from build123d import *

# Parameters (mm, degrees)
F3_DEPTH = 9
F4_SIZE  = 1


with BuildPart() as f1:
    # F0 (on Top) → F1 (revolve)
    with BuildSketch(Plane.XY):
        Polygon((-4, 0), (0, 0), (0, 41), (-6.5, 41), (-6.5, 30), (-4, 30), align=None)
    revolve(axis=Axis((0, 20.5, 0), (0, 1, 0)))

    # F2 (on face) → F3 (cut)
    with BuildSketch(Plane(origin=(0, 41, 0), x_dir=(-1, 0, 0), z_dir=(0, 1, 0))):
        Polygon((-3.255243, -1.184649), (-0.601686, -3.411448), (2.653557, -2.226799), (3.255243, 1.184649), (0.601686, 3.411448), (-2.653557, 2.226799), align=None)
    extrude(amount=-F3_DEPTH, mode=Mode.SUBTRACT)

    # F4
    f4_edges = [f1.edges().sort_by_distance(p)[0] for p in [
        (6.5, 41, 0),
    ]]
    chamfer(f4_edges, length=F4_SIZE)


solid = f1.part
Build history of the part. All positions in model axes, mm. A direction names the side the tool comes from. Coordinates: 2 decimals unless noted, no trailing zeros. Write each loop counter-clockwise with the first axis right and the second up, starting at its lowest first coordinate (ties: lowest second). Pieces come first, ordered by that corner, then holes.
(1) Drill centre lines: line 1 (X direction, y = 9, z = -3); line 2 (Y direction, x = -1.75, z = 2); line 3 (X direction, y = 35.5, z = 1). Where is each one in solid material? Low to high.
(2) Cut at D-D on y = 20. List the corners of the cut face in (x, z).
(3) Cut at B-B on z = 0. List the corners of the cut face in (x, y).
(4) Cut at C-C on x = 0. List the corners of the cut face in (y, z), and give its area (3 significant figures).
(5) 3-axis set-ups, long thin cutter, end or side, ignore diameter. For faces 5 (the flat face through (2.95, 36.56, 0.54)), 6 (the flat face through (-3, 30, 3)), 7 (the cylindrical face through (5.158, 34.93, -3.955)): which of +Z, -Z, +X, -X, +Y, -Y reach the whole face in a straight line?
(6) Mould opens along Z. For faces 1 (the flat face through (1.95, 36.56, -2.28)), 2 (the flat face through (2.4, 41, -2.4)), 3 (the flat face through (0, 32, 0)), 4 (the cylindrical face through (0.867, 14.79, -3.905)) say: pulls with the +Z half, pulls with the -Z half, needs draft (parallel to the pull), parting line crosses it, or undercut.
(7) Cut at A-A on y = 36. List the corners of the cut face in (x, z).
(8) Pin check, flat tips, straight feed: pin 1 Ø3 at (x, y) = (-5, 35) entering from +Z; pin 2 Ø4 at (y, z) = (16, -1.5) entering from +X. Stop position of each tip, or through.
Working result:
1. line 1: x = -2.65 to 2.65
1. line 2: y = 0 to 32
1. line 3: x = -6.42 to -3.22, 2.87 to 6.42
2. outline: circle Ø8 at (0, 0)
3. outline: (-6.5, 30) - (-4, 30) - (-4, 0) - (4, 0) - (4, 30) - (6.5, 30) - (6.5, 40) - (5.5, 41) - (3.05, 41) - (3.05, 32) - (-3.05, 32) - (-3.05, 41) - (-5.5, 41) - (-6.5, 40) - close
4. outline: (0, -4) - (30, -4) - (30, -6.5) - (40, -6.5) - (41, -5.5) - (41, -3.19) - (32, -3.19) - (32, 3.19) - (41, 3.19) - (41, 5.5) - (40, 6.5) - (30, 6.5) - (30, 4) - (0, 4) - close
4. area: 325 mm2
5. face 5: +Y
5. face 6: -Y
5. face 7: +Y, -Y
6. face 1: undercut
6. face 2: needs draft
6. face 3: undercut
6. face 4: parting line crosses it
7. outline: circle Ø13 at (0, 0); hole (-3.26, 1.18) - (-2.65, -2.23) - (0.6, -3.41) - (3.26, -1.18) - (2.65, 2.23) - (-0.6, 3.41) - close
8. pin 1: stops at z = 5.48
8. pin 2: stops at x = 4
